```python
from build123d import *

# Parameters (mm, degrees)
SKETCH_1_W      = 70
SKETCH_1_H      = 8
EXTRUDE_1_DEPTH = 2
FILLET_1_R      = 3.4


with BuildPart() as part:
    # 草图1 → 凸台-拉伸1 (new body)
    with BuildSketch(Plane(origin=(0, 0, 0), x_dir=(1, 0, 0), z_dir=(0, 1, 0))):
        Rectangle(SKETCH_1_W, SKETCH_1_H)
        with BuildLine():
            ThreePointArc((-30, -1.7), (-31.7, 0), (-30, 1.7))
            Line((-30, 1.7), (30, 1.7))
            ThreePointArc((30, 1.7), (31.202081528, 1.202081528), (31.7, 0))
            ThreePointArc((31.7, 0), (31.202081528, -1.202081528), (30, -1.7))
            Line((30, -1.7), (-30, -1.7))
        make_face(mode=Mode.SUBTRACT)
    extrude(amount=EXTRUDE_1_DEPTH)

    # 圆角1
    fillet_1_edges = [part.edges().sort_by_distance(p)[0] for p in [
        (35, 1, 4),
        (-35, 1, 4),
        (-35, 1, -4),
        (35, 1, -4),
    ]]
    fillet(fillet_1_edges, radius=FILLET_1_R)


solid = part.part
```
Verification items for the finished model (mm, model axes). A direction names the side the tool comes from. Round coordinates to 2 decimals unless told otherwise and drop trailing zeros. Order: outer loops, then holes, each group sorted by start corner. A loop starts at its lowest first (then second) coordinate and runs counter-clockwise, first axis right, second up.
1) Material ranges on line 1 (Z direction, x = 28, y = 0.25); line 2 (X direction, y = 0.15, z = -0.5); line 3 (X direction, y = 0.2, z = 1), recorded low to high.
Geometry says:
line 1: z = -4 to -1.7, 1.7 to 4
line 2: x = -35 to -31.62, 31.62 to 35
line 3: x = -34.98 to -31.37, 31.37 to 34.98
2) Cross-section at A-A, the plane y = 1.35. Record the cut outline in (x, z), plus the area to 3 significant figures.
Geometry says:
outline: (-35, -0.6) arc R3.4 ccw to (-31.6, -4) - (31.6, -4) arc R3.4 ccw to (35, -0.6) - (35, 0.6) arc R3.4 ccw to (31.6, 4) - (-31.6, 4) arc R3.4 ccw to (-35, 0.6) - close; hole (-30, -1.7) - (30, -1.7) arc R1.7 ccw to (30, 1.7) - (-30, 1.7) arc R1.7 ccw to start
area: 337 mm2
3) Tool access check on faces 1 (the flat face through (0, 1, -1.7)), 2 (the cylindrical face through (-34.03, 1.01, -2.98)). Record the directions out of +Z, -Z, +X, -X, +Y, -Y that give a thin tool (end or side, any length) a straight path to the whole face; none if there is none.
Geometry says:
face 1: +Y, -Y
face 2: -Z, -X, +Y, -Y
4) Cross-section at B-B, the plane x = -26. Record the cut outline in (y, z).
Geometry says:
outline: (0, -4) - (2, -4) - (2, -1.7) - (0, -1.7) - close; (0, 1.7) - (2, 1.7) - (2, 4) - (0, 4) - close
5) Cross-section at C-C, the plane z = 3. Record the cut outline in (x, y), plus the area to 3 significant figures.
Geometry says:
outline: (-34.01, 0) - (34.01, 0) - (34.01, 2) - (-34.01, 2) - close
area: 136 mm2
6) Draft check along X on faces 3 (the flat face through (35, 1, 0)), 4 (the cylindrical face through (-31.7, 1, 0)), 5 (the flat face through (0, 1, -4)). Enter one of: +X half, -X half, draft (parallel to the pull), parting line (faces both ways), or undercut.
Geometry says:
face 3: +X half
face 4: undercut
face 5: draft
